Source: CAD feature listing. Evaluate the final solid. Frame: model axes, mm. A direction names the side the tool comes from. Coordinates: 2 decimals unless noted, no trailing zeros. Loops run counter-clockwise (first coordinate to the right, second up) from the corner with the lowest first, then second, coordinate; pieces in that order, holes last.
Item 1: Section query A-A, the plane z = -101.6. Return the cut outline in (x, y) (3 decimals).
Item 2: Reachability of faces 1 (the flat face through (57, 52, -151.6)), 2 (the flat face through (60.55, 64, -113)), 3 (the cylindrical face through (15.24, 1.61, -33.74)) from +Z, -Z, +X, -X, +Y, -Y: full face, straight path, thin tool, end or side. Return the list, or none.
Item 3: Pin query (flat end, axial travel): pin 1 Ø3 at (x, y) = (58, 72.5) entering from -Z; pin 2 Ø5 at (y, z) = (40.56, -79.76) entering from -X; pin 3 Ø5 at (y, z) = (68, -86.5) entering from +X; pin 4 Ø3.5 at (y, z) = (1, -86) entering from -X. Return the tip coordinate at first contact, or that it passes through.
Item 4: Section query C-C, the plane x = 36.5. Return the cut outline in (y, z) (3 decimals).
Item 5: Line query: probe 1 along Y at (x, z) = (57, -101) (3 decimals); probe 2 along Y at (x, z) = (38, -121.5) (3 decimals); probe 3 along X at (y, z) = (82, -99.5). Output: solid intervals per line, ascending.
Item 6: Pull-direction query (Z, two-part tool) for faces 4 (the cylindrical face through (150.12, 1.61, -33.74)), 5 (the flat face through (54.2, 64, -113)), 6 (the flat face through (57, 52, -51.6)); classes: +Z half, -Z half, draft (parallel to the pull), parting line (faces both ways), or undercut.
Item 7: Section query D-D, the plane y = 12.5. Return the cut outline in (x, z).
Item 8: Section query B-B, the plane z = -62. Return the cut outline in (x, y) (3 decimals).
```python
from build123d import *

# Parameters (mm, degrees)
SKETCH1_W                = 165.1
SKETCH1_H                = 203.2
BOSS_EXTRUDE1_DEPTH      = 3.175
CUT_EXTRUDE1_DEPTH       = 4.175
SKETCH3_W                = 6.35
SKETCH3_H                = 100
BOSS_EXTRUDE2_DEPTH      = 100
F_6_0_6_DIAMETER_HOLE1_D = 6
SKETCH4_R                = 12.7
CUT_EXTRUDE2_DEPTH       = 61.549652809


with BuildPart() as part:
    # Sketch1 → Boss-Extrude1 (new body)
    with BuildSketch(Plane(origin=(0, 0, 0), x_dir=(1, 0, 0), z_dir=(0, 1, 0))):
        with Locations((82.55, 101.6)):
            Rectangle(SKETCH1_W, SKETCH1_H)
    extrude(amount=BOSS_EXTRUDE1_DEPTH)

    # Sketch2 → Cut-Extrude1 (cut, through all)
    with BuildSketch(Plane(origin=(0, 3.175, 0), x_dir=(-1, 0, 0), z_dir=(0, 1, 0))):
        with BuildLine():
            Line((-9.113, -39.738854308), (-9.113, -163.461145692))
            ThreePointArc((-9.113, -163.461145692), (-15.113, -169.461145692), (-21.113, -163.461145692))
            Line((-21.113, -163.461145692), (-21.113, -39.738854308))
            ThreePointArc((-21.113, -39.738854308), (-15.113, -33.738854308), (-9.113, -39.738854308))
        make_face()
        with BuildLine():
            Line((-143.987, -39.738854308), (-143.987, -163.461145692))
            ThreePointArc((-143.987, -163.461145692), (-149.987, -169.461145692), (-155.987, -163.461145692))
            Line((-155.987, -163.461145692), (-155.987, -39.738854308))
            ThreePointArc((-155.987, -39.738854308), (-149.987, -33.738854308), (-143.987, -39.738854308))
        make_face()
    extrude(amount=-CUT_EXTRUDE1_DEPTH, mode=Mode.SUBTRACT)

    # Sketch3 → Boss-Extrude2 (add)
    with BuildSketch(Plane(origin=(0, 3.175, 0), x_dir=(-1, 0, 0), z_dir=(0, 1, 0))):
        with Locations((-57.374652809, -101.6)):
            Rectangle(SKETCH3_W, SKETCH3_H)
    extrude(amount=BOSS_EXTRUDE2_DEPTH)

    # Ø6.0 (6) Diameter Hole1 (through all)
    with Locations(Plane(origin=(60.549652809, 78.39827856, -101.6), x_dir=(0, 0, 1), z_dir=(1, 0, 0))):
        with Locations((0, 0), (21.844, 37.83491784), (-21.844, 37.83491784)):
            Hole(F_6_0_6_DIAMETER_HOLE1_D / 2)

    # Sketch4 → Cut-Extrude2 (cut, through all)
    with BuildSketch(Plane(origin=(60.549652809, 0, 0), x_dir=(0, 0, -1), z_dir=(1, 0, 0))):
        with Locations((101.6, 53.175)):
            Circle(SKETCH4_R)
    extrude(amount=-CUT_EXTRUDE2_DEPTH, mode=Mode.SUBTRACT)


solid = part.part
```
Verdict:
1. outline: (0, 0) - (9.113, 0) - (9.113, 3.175) - (0, 3.175) - close; (21.113, 0) - (143.987, 0) - (143.987, 3.175) - (60.55, 3.175) - (60.55, 40.475) - (54.2, 40.475) - (54.2, 3.175) - (21.113, 3.175) - close; (54.2, 65.875) - (60.55, 65.875) - (60.55, 75.398) - (54.2, 75.398) - close; (54.2, 81.398) - (60.55, 81.398) - (60.55, 103.175) - (54.2, 103.175) - close; (155.987, 0) - (165.1, 0) - (165.1, 3.175) - (155.987, 3.175) - close
2. face 1: -Z, +X, -X, +Y
2. face 2: +Z, -Z, +X, +Y
2. face 3: +Y, -Y
3. pin 1: stops at z = -151.6
3. pin 2: passes through
3. pin 3: stops at x = 60.55
3. pin 4: stops at x = 0
4. outline: (0, -203.2) - (3.175, -203.2) - (3.175, 0) - (0, 0) - close
5. probe 1: y = 0 to 40.489, 65.861 to 75.459, 81.338 to 103.175
5. probe 2: y = 0 to 3.175
5. probe 3: x = 54.2 to 60.55
6. face 4: undercut
6. face 5: draft
6. face 6: +Z half
7. outline: (54.2, -151.6) - (60.55, -151.6) - (60.55, -51.6) - (54.2, -51.6) - close
8. outline: (0, 0) - (9.113, 0) - (9.113, 3.175) - (0, 3.175) - close; (21.113, 0) - (143.987, 0) - (143.987, 3.175) - (60.55, 3.175) - (60.55, 103.175) - (54.2, 103.175) - (54.2, 3.175) - (21.113, 3.175) - close; (155.987, 0) - (165.1, 0) - (165.1, 3.175) - (155.987, 3.175) - close
